For this review, use the dimensioned drawing (mm, ordinates from the lowest corner) and the shaded views. A direction names the side the tool comes from. Give positions to 0.01 mm unless a question says otherwise; leave off trailing zeros. Order: outer loops, then holes, each group sorted by start corner. A loop starts at its lowest first (then second) coordinate and runs counter-clockwise, first axis right, second up.
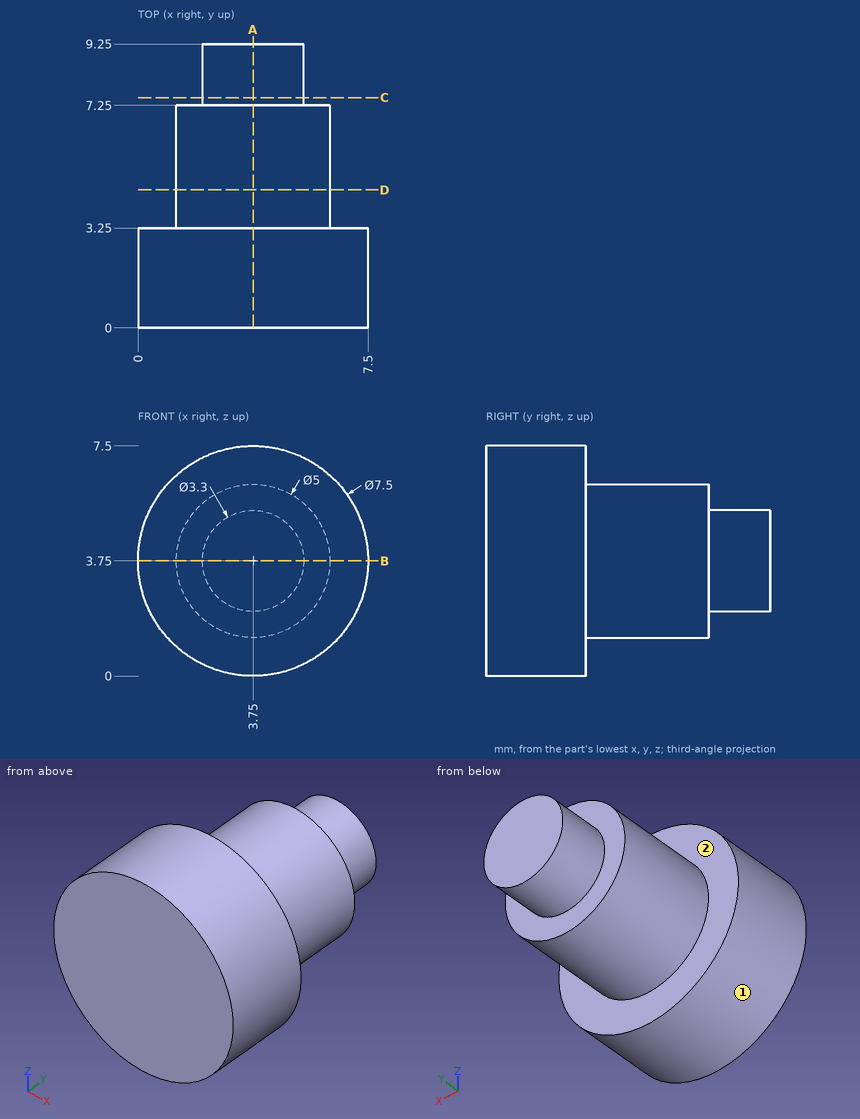
1. Take a section at B-B (z = 3.75). Write out the cut boundary in (x, y), and give its area (3 significant figures).
2. Take a section at A-A (x = 3.75). Write out the cut boundary in (y, z).
3. For the marked faces 1 and 2, list the 3-axis set-ups (+Z, -Z, +X, -X, +Y, -Y) from which the entire face can be reached by the end or side of a thin tool; tool diameter is ignored.
4. Take a section at D-D (y = 4.5). Write out the cut boundary in (x, z), and give its area (3 significant figures).
5. Take a section at C-C (y = 7.5). Write out the cut boundary in (x, z), and give its area (3 significant figures).
6. Insertion check: pin 1 (2 mm diameter, centred on y = 5, z = 4, fed in from -X); pin 2 (1 mm diameter, centred on y = 6.5, z = 4, fed in from +X); pin 3 (2 mm diameter, centred on x = 5.5, y = 8, fed in from +Z). Each pin has a flat end and moves straight along its axis. Give the tip position at first contact, or say it passes through.
7. To check wall thickness, follow line 1 (Y direction, x = 5, z = 6.5); line 2 (Y direction, x = 2, z = 2); line 3 (X direction, y = 3, z = 3.25). State the ranges of each line that lie inside material, in increasing order.
Answer:
1. outline: (0, 0) - (7.5, 0) - (7.5, 3.25) - (6.25, 3.25) - (6.25, 7.25) - (5.4, 7.25) - (5.4, 9.25) - (2.1, 9.25) - (2.1, 7.25) - (1.25, 7.25) - (1.25, 3.25) - (0, 3.25) - close
1. area: 51.0 mm2
2. outline: (0, 0) - (3.25, 0) - (3.25, 1.25) - (7.25, 1.25) - (7.25, 2.1) - (9.25, 2.1) - (9.25, 5.4) - (7.25, 5.4) - (7.25, 6.25) - (3.25, 6.25) - (3.25, 7.5) - (0, 7.5) - close
3. face 1: +Y, -Y
3. face 2: +Y
4. outline: circle Ø5 at (3.75, 3.75)
4. area: 19.6 mm2
5. outline: circle Ø3.3 at (3.75, 3.75)
5. area: 8.55 mm2
6. pin 1: stops at x = 1.25
6. pin 2: stops at x = 6.25
6. pin 3: stops at z = 6
7. line 1: y = 0 to 3.25
7. line 2: y = 0 to 7.25
7. line 3: x = 0.03 to 7.47
